Source: CAD feature listing. Evaluate the final solid. Frame: model axes, mm. Face numbers are marked on the shaded views. A direction names the side the tool comes from. Give positions to 0.01 mm unless a question says otherwise; leave off trailing zeros. Order: outer loops, then holes, each group sorted by start corner. A loop starts at its lowest first (then second) coordinate and runs counter-clockwise, first axis right, second up.
1) Material intervals for line 1 (Z direction, x = 76.35, y = 93); line 2 (X direction, y = 106, z = 80); line 3 (X direction, y = -1, z = -90), sorted ascending.
2) Draft query along X for the marked faces 1, 2 and 3. Return one class per face: released by +X, released by -X, zero draft, split by the parting line, or undercut.
3) Section A-A, the plane y = 93. Return loops of the section in (x, z).
4) First-contact query: P1, Ø2, axis at x = 33, z = 54.5, coming from the +Y side; P2, Ø9, axis at x = -47, z = -90, coming from the +Y side; P3, Ø16, axis at x = 47, z = 90, coming from the -Y side; P4, Ø1.5, axis at y = 4.94, z = 52.53, coming from the -X side. Flat tips, straight axial feed; report the tip coordinate or a pass-through.
5) Access query for the marked faces 4 and 5. Directions: +Z, -Z, +X, -X, +Y, -Y. A direction counts if a zero-diameter tool reaches every point of the face in a straight line with its end or side. Return the directions, or none.
6) Section D-D, the plane z = -90. Return loops of the section in (x, y) (3 decimals), plus the area to 3 significant figures.
7) Section B-B, the plane z = -10. Return loops of the section in (x, y), plus the area to 3 significant figures.
8) Section C-C, the plane y = 28. Return loops of the section in (x, z), plus the area to 3 significant figures.
```python
from build123d import *

# Parameters (mm, degrees)
SKETCH1_W                      = 150
SKETCH1_H                      = 230
BASE_FLANGE1_DEPTH             = 2
EDGE_FLANGE1_STRIP_W           = 28
EDGE_FLANGE1_STRIP_H           = 2
EDGE_FLANGE1_STRIP_CUT_DEPTH   = 230
EDGE_FLANGE1_STRIP_2_W         = 28
EDGE_FLANGE1_STRIP_2_H         = 2
EDGE_FLANGE1_STRIP_CUT_2_DEPTH = 230
EDGE_FLANGE1_DEPTH             = 230
EDGE_FLANGE1_BEND_DEPTH        = 230
SKETCH15_OUTSIDE_W             = 298.254
SKETCH15_OUTSIDE_H             = 250.254
SKETCH15_OUTSIDE_R             = 8
CUT_EXTRUDE1_DEPTH             = 264.326793168
SKETCH16_R                     = 5
CUT_EXTRUDE2_DEPTH             = 228.055059487
CUT_EXTRUDE3_DEPTH             = 228.055059487
SKETCHED_START                 = 47
SKETCHED_BEND1_DEPTH           = 11.052994728
SKETCHED_BEND1_2_DEPTH         = 11.052994728
CUT_EXTRUDE4_REACH             = 241.866
SKETCH20_R                     = 1.25


# Read off the part's stored shape, not the designer's step: Sketched Bend1
# Sheet-metal steps are written as plain solids
with BuildPart() as part:
    # Sketch1 → Base-Flange1 (new body)
    with BuildSketch(Plane(origin=(0, 0, 0), x_dir=(1, 0, 0), z_dir=(0, 1, 0))):
        Rectangle(SKETCH1_W, SKETCH1_H)
    extrude(amount=-BASE_FLANGE1_DEPTH)

    # Edge-Flange1 strip (across the edge) → Edge-Flange1 strip cut (cut)
    with BuildSketch(Plane(origin=(75, 0, 115), x_dir=(-1, 0, 0), z_dir=(0, 0, -1))):
        with Locations((-4, -1)):
            Rectangle(EDGE_FLANGE1_STRIP_W, EDGE_FLANGE1_STRIP_H)
    extrude(amount=EDGE_FLANGE1_STRIP_CUT_DEPTH, mode=Mode.SUBTRACT)

    # Edge-Flange1 strip 2 (across the edge) → Edge-Flange1 strip cut 2 (cut)
    with BuildSketch(Plane(origin=(-75, 0, -115), x_dir=(1, 0, 0), z_dir=(0, 0, 1))):
        with Locations((-4, -1)):
            Rectangle(EDGE_FLANGE1_STRIP_2_W, EDGE_FLANGE1_STRIP_2_H)
    extrude(amount=EDGE_FLANGE1_STRIP_CUT_2_DEPTH, mode=Mode.SUBTRACT)

    # Edge-Flange1 section (across the edge) → Edge-Flange1 (add)
    with BuildSketch(Plane(origin=(75, 0, 115), x_dir=(-1, 0, 0), z_dir=(0, 0, -1))):
        with BuildLine():
            Line((-2, 10), (-2, 180))
            Line((-2, 180), (0, 180))
            Line((0, 180), (0, 10))
            ThreePointArc((0, 10), (2.928932188, 2.928932188), (10, 0))
            Line((10, 0), (10, -2))
            ThreePointArc((10, -2), (1.514718626, 1.514718626), (-2, 10))
        make_face()
    extrude(amount=EDGE_FLANGE1_DEPTH)

    # Edge-Flange1 section 2 (across the edge) → Edge-Flange1 bend (add)
    with BuildSketch(Plane(origin=(-75, 0, -115), x_dir=(1, 0, 0), z_dir=(0, 0, 1))):
        with BuildLine():
            Line((-2, 10), (-2, 180))
            Line((-2, 180), (0, 180))
            Line((0, 180), (0, 10))
            ThreePointArc((0, 10), (2.928932188, 2.928932188), (10, 0))
            Line((10, 0), (10, -2))
            ThreePointArc((10, -2), (1.514718626, 1.514718626), (-2, 10))
        make_face()
    extrude(amount=EDGE_FLANGE1_BEND_DEPTH)

    # Sketch15 outside → Cut-Extrude1 (cut, through all)
    # profile 1 of 4: a face of its own
    with BuildSketch(Plane.ZY.offset(77)):
        with Locations((0, 89)):
            Rectangle(SKETCH15_OUTSIDE_W, SKETCH15_OUTSIDE_H)
        with BuildLine():
            Line((21.083470393, 171.180744276), (96.507242037, 119.243178795))
            ThreePointArc((96.507242037, 119.243178795), (101.277963521, 113.867184852), (103, 106.888955512))
            Line((103, 106.888955512), (103, 16))
            ThreePointArc((103, 16), (104.757359313, 11.757359313), (109, 10))
            Line((109, 10), (110, 10))
            ThreePointArc((110, 10), (113.535533906, 8.535533906), (115, 5))
            Line((115, 5), (115, -2))
            Line((115, -2), (-115, -2))
            Line((-115, -2), (-115, 99))
            Line((-115, 99), (-115, 150))
            ThreePointArc((-115, 150), (-106.213203436, 171.213203436), (-85, 180))
            Line((-85, 180), (-49, 180))
            Line((-49, 180), (-7.274003064, 180))
            ThreePointArc((-7.274003064, 180), (7.574612801, 177.744304445), (21.083470393, 171.180744276))
        make_face(mode=Mode.SUBTRACT)
    # profile 2 of 4: a face of its own
    with BuildSketch(Plane.ZY.offset(77)):
        with Locations(Location((50, 93, 0), (0, 0, 270))):
            Circle(SKETCH15_OUTSIDE_R)
    # profile 3 of 4: a face of its own
    with BuildSketch(Plane.ZY.offset(77)):
        with Locations(Location((-85, 150, 0), (0, 0, 270))):
            Circle(SKETCH15_OUTSIDE_R)
    # profile 4 of 4: a face of its own
    with BuildSketch(Plane.ZY.offset(77)):
        with Locations(Location((-10, 65, 0), (0, 0, 270))):
            Circle(SKETCH15_OUTSIDE_R)
    extrude(amount=-CUT_EXTRUDE1_DEPTH, mode=Mode.SUBTRACT)

    # Sketch16 → Cut-Extrude2 (cut, through all)
    with BuildSketch(Plane(origin=(0, 0, 0), x_dir=(1, 0, 0), z_dir=(0, 1, 0))):
        with Locations(Location((-47, 90, 0), (0, 0, 270))):
            Circle(SKETCH16_R)
        with Locations(Location((47, 90, 0), (0, 0, 90))):
            Circle(SKETCH16_R)
        with Locations(Location((47, -90, 0), (0, 0, 270))):
            Circle(SKETCH16_R)
        with Locations(Location((-47, -90, 0), (0, 0, 90))):
            Circle(SKETCH16_R)
        with BuildLine():
            Line((7.5, 20), (7.5, -20))
            ThreePointArc((7.5, -20), (0, -27.5), (-7.5, -20))
            Line((-7.5, -20), (-7.5, 20))
            ThreePointArc((-7.5, 20), (0, 27.5), (7.5, 20))
        make_face()
    extrude(amount=-CUT_EXTRUDE2_DEPTH, mode=Mode.SUBTRACT)

    # Sketch18 → Cut-Extrude3 (cut, through all)
    with BuildSketch(Plane(origin=(0, 0, 0), x_dir=(1, 0, 0), z_dir=(0, 1, 0))):
        Polygon((31.4, -45), (44.4, -45), (44.4, -60.052994728), (31.4, -60.052994728), (31.4, -58.052994728), (42.4, -58.052994728), (42.4, -47), (31.4, -47), align=None)
    extrude(amount=-CUT_EXTRUDE3_DEPTH, mode=Mode.SUBTRACT)

    # Sketched Bend1 outline → Sketched Bend1 (cut)
    with BuildSketch(Plane.XY.offset(SKETCHED_START)):
        with BuildLine():
            ThreePointArc((34.035602398, 0), (33.054267209, -1.443395312), (31.4, -2))
            Line((31.4, -2), (42.4, -2))
            Line((42.4, -2), (42.4, 0))
            Line((42.4, 0), (34.035602398, 0))
        make_face()
    extrude(amount=SKETCHED_BEND1_DEPTH, mode=Mode.SUBTRACT)

    # Sketched Bend1 2 outline → Sketched Bend1 2 (add)
    with BuildSketch(Plane.XY.offset(SKETCHED_START)):
        with BuildLine():
            Line((31.4, 0), (34.035602398, 0))
            ThreePointArc((34.035602398, 0), (34.111233029, 0.364854094), (34.1366, 0.7366))
            Line((34.1366, 0.7366), (34.1366, 9.008755099))
            Line((34.1366, 9.008755099), (32.1366, 9.008755099))
            Line((32.1366, 9.008755099), (32.1366, 0.7366))
            ThreePointArc((32.1366, 0.7366), (31.920854855, 0.215745145), (31.4, 0))
        make_face()
    extrude(amount=SKETCHED_BEND1_2_DEPTH)

    # Sketch20 → Cut-Extrude4 (cut, up to next)
    with BuildSketch(Plane.ZY.offset(-32.1366), mode=Mode.PRIVATE) as cut_extrude4_sk1:
        with Locations(Location((52.526497364, 4.9366, 0), (0, 0, 270))):
            Circle(SKETCH20_R)
    cut_extrude4_tool1 = extrude(cut_extrude4_sk1.sketch, amount=-CUT_EXTRUDE4_REACH, mode=Mode.PRIVATE) & part.part
    add(cut_extrude4_tool1.solids().sort_by_distance((32.1366, 4.9366, 52.526497))[0], mode=Mode.SUBTRACT)


solid = part.part
```
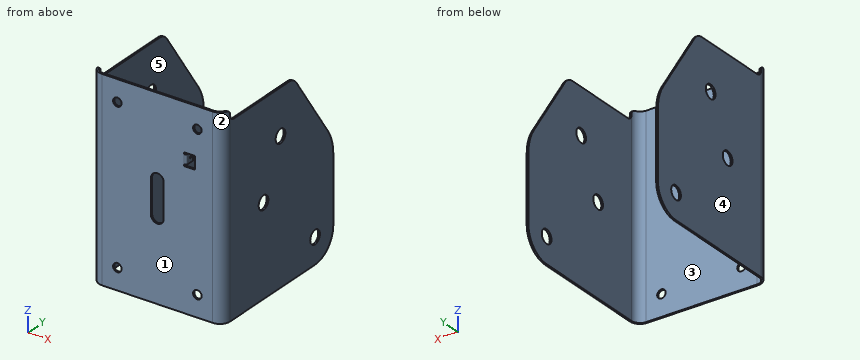
From the geometry:
1. line 1: z = -115 to 42, 58 to 103
1. line 2: x = -77 to -75, 75 to 77
1. line 3: x = -69.8 to -52, -42 to 42, 52 to 69.8
2. face 1: zero draft
2. face 2: released by +X
2. face 3: undercut
3. outline: (-77, -115) - (-75, -115) - (-75, 42) - (-77, 42) - close; (-77, 58) - (-75, 58) - (-75, 103) - (-77, 103) - close; (75, -115) - (77, -115) - (77, 42) - (75, 42) - close; (75, 58) - (77, 58) - (77, 103) - (75, 103) - close
4. P1: stops at y = 9.01
4. P2: passes through
4. P3: stops at y = -2
4. P4: stops at x = -76.2
5. face 4: +Z, -Z, -X, +Y, -Y
5. face 5: +Z, -Z, +Y
6. outline: (-77, 10) arc R12 ccw to (-65, -2) - (-52, -2) - (-52, 0) - (-65, 0) arc R10 cw to (-75, 10) - (-75, 143.755) - (-77, 143.755) - close; (-77, 156.245) - (-75, 156.245) - (-75, 179.58) - (-77, 179.58) - close; (-42, -2) - (42, -2) - (42, 0) - (-42, 0) - close; (52, -2) - (65, -2) arc R12 ccw to (77, 10) - (77, 143.755) - (75, 143.755) - (75, 10) arc R10 cw to (65, 0) - (52, 0) - close; (75, 156.245) - (77, 156.245) - (77, 179.58) - (75, 179.58) - close
6. area: 917 mm2
7. outline: (-77, 10) arc R12 ccw to (-65, -2) - (-7.5, -2) - (-7.5, 0) - (-65, 0) arc R10 cw to (-75, 10) - (-75, 57) - (-77, 57) - close; (-77, 73) - (-75, 73) - (-75, 180) - (-77, 180) - close; (7.5, -2) - (65, -2) arc R12 ccw to (77, 10) - (77, 57) - (75, 57) - (75, 10) arc R10 cw to (65, 0) - (7.5, 0) - close; (75, 73) - (77, 73) - (77, 180) - (75, 180) - close
7. area: 915 mm2
8. outline: (-77, -115) - (-75, -115) - (-75, 103) - (-77, 103) - close; (75, -115) - (77, -115) - (77, 103) - (75, 103) - close
8. area: 872 mm2
